The figure shows three views and two pictorial views of one solid part (mm, origin at its lowest corner). Answer the questions. A direction names the side the tool comes from. Give positions to 0.01 mm unless a question says otherwise; leave off trailing zeros. Loops run counter-clockwise (first coordinate to the right, second up) from the corner with the lowest first, then second, coordinate; pieces in that order, holes last. Notation, with made-up numbers: M -2,-38 L 15,-38 A27 cw 15,-20 Z; hole C -25.75,51 d5. An arc over 180 degrees is marked long. Write item = value, one per line. Start each with the question number.
1. Section A-A on x = 3 is taken. Determine the outline of the cut face in (y, z), plus the area to 3 significant figures.
2. For the marked faces 1, 2, 3 and 4, determine the directions among +Z, -Z, +X, -X, +Y, -Y from which every point of the face is accessible in a straight line to the end or side of a thin tool.
3. Flat-ended cylindrical pins translate along their axes: pin 1 Ø3 at (x, z) = (3.5, 21) entering from -Y; pin 2 Ø10 at (x, z) = (31, 4) entering from -Y; pin 3 Ø6 at (x, y) = (12.5, 22) entering from +Z; pin 4 Ø4 at (x, z) = (9.5, 20) entering from -Y. Find the tip coordinate at first contact, or state that the pin passes through.
4. Consider L1, parallel to Z at x = 8, y = 3.75; L2, parallel to X at y = 1.5, z = 1.5; L3, parallel to X at y = 20, z = 16.5. Determine where each line is inside the solid, lowest interval first. Write a range as [from, to].
5. Section D-D on z = 18.75 is taken. Determine the outline of the cut face in (x, y).
6. Section B-B on z = 10.75 is taken. Determine the outline of the cut face in (x, y), plus the area to 3 significant figures.
7. Section C-C on y = 2.5 is taken. Determine the outline of the cut face in (x, z), plus the area to 3 significant figures.
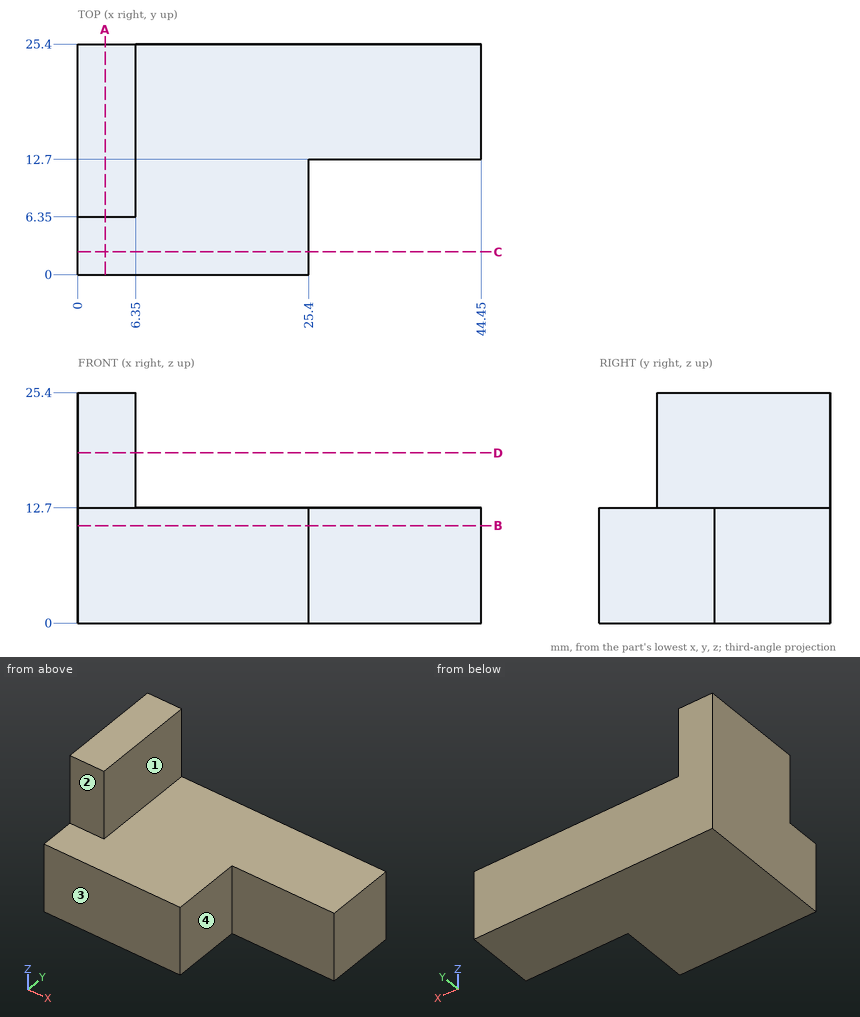
Verdict:
q1.outline = M 0,0 L 25.4,0 L 25.4,25.4 L 6.35,25.4 L 6.35,12.7 L 0,12.7 Z
q1.area = 565 mm2
q2.face_1 = +Z, +X, +Y, -Y
q2.face_2 = +Z, +X, -X, -Y
q2.face_3 = +Z, -Z, +X, -X, -Y
q2.face_4 = +Z, -Z, +X, -Y
q3.pin_1 = 6.35
q3.pin_2 = 12.7
q3.pin_3 = 12.7
q3.pin_4 = through
q4.L1 = [0, 12.7]
q4.L2 = [0, 25.4]
q4.L3 = [0, 6.35]
q5.outline = M 0,6.35 L 6.35,6.35 L 6.35,25.4 L 0,25.4 Z
q6.outline = M 0,0 L 25.4,0 L 25.4,12.7 L 44.45,12.7 L 44.45,25.4 L 0,25.4 Z
q6.area = 887 mm2
q7.outline = M 0,0 L 25.4,0 L 25.4,12.7 L 0,12.7 Z
q7.area = 323 mm2
